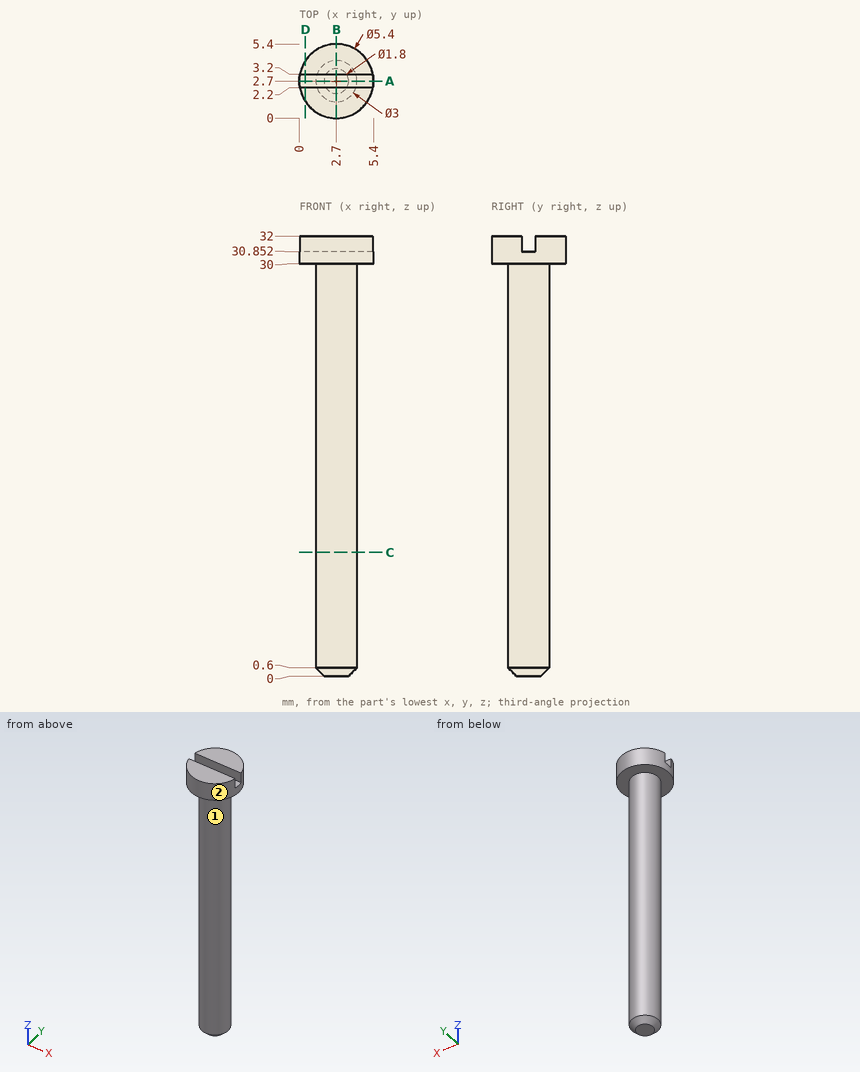
Geometry: see drawing. Coordinates: mm, zero at the bounding-box minimum. A direction names the side the tool comes from. Coordinates: 2 decimals unless noted, no trailing zeros. Order: outer loops, then holes, each group sorted by start corner. A loop starts at its lowest first (then second) coordinate and runs counter-clockwise, first axis right, second up. Notation, with made-up numbers: M 76,-15 L 134,-15 A18 ccw 134,12 Z; hole C -0.75,-1 d11. An arc over 180 degrees is marked long. Answer in a Markdown table with one row per item. Add a question column.
Q1. Section query D-D on x = 0.45. Return the cut outline in (y, z).
Q2. Section query A-A on y = 2.7. Return the cut outline in (x, z), and give its area (3 significant figures).
Q3. Line query: L1, parallel to Z at x = 2.7, y = 1.75; L2, parallel to X at y = 2.8, z = 12. Output: solid intervals per line, ascending.
Q4. Section query B-B on x = 2.7. Return the cut outline in (y, z).
Q5. Contact query for flat-ended pins moving along their axis: P1, Ø1, axis at y = 4.5, z = 17, coming from the +X side; P2, Ø1.5, axis at x = 2, z = 19.5, coming from the +Y side; P3, Ø3, axis at x = 0.5, y = 1.5, coming from the -Z side. Output: stop coordinate, or through.
Q6. Reachability of the marked faces 1 and 2 from +Z, -Z, +X, -X, +Y, -Y: full face, straight path, thin tool, end or side. Return the list, or none.
Q7. Section query C-C on z = 9. Return the cut outline in (x, y).
Completed:
| question | item | result |
|---|---|---|
| 1 | outline | M 1.21,30 L 4.19,30 L 4.19,32 L 3.2,32 L 3.2,30.85 L 2.2,30.85 L 2.2,32 L 1.21,32 Z |
| 2 | outline | M 0,30 L 1.2,30 L 1.2,0.6 L 1.8,0 L 3.6,0 L 4.2,0.6 L 4.2,30 L 5.4,30 L 5.4,30.85 L 0,30.85 Z |
| 2 | area | 94.2 mm2 |
| 3 | L1 | z = 0.05 to 32 |
| 3 | L2 | x = 1.2 to 4.2 |
| 4 | outline | M 0,30 L 1.2,30 L 1.2,0.6 L 1.8,0 L 3.6,0 L 4.2,0.6 L 4.2,30 L 5.4,30 L 5.4,32 L 3.2,32 L 3.2,30.85 L 2.2,30.85 L 2.2,32 L 0,32 Z |
| 5 | P1 | stops at x = 3.45 |
| 5 | P2 | stops at y = 4.2 |
| 5 | P3 | stops at z = 0.11 |
| 6 | face 1 | -Z |
| 6 | face 2 | +Z, -Z |
| 7 | outline | C 2.7,2.7 d3 |
